Input: part model. Units: mm. Frame: model coordinates. A direction names the side the tool comes from. Coordinates: 2 decimals unless noted, no trailing zeros. Loops run counter-clockwise (first coordinate to the right, second up) from the corner with the lowest first, then second, coordinate; pieces in that order, holes last.
Autodesk Inventor part; units mm, degrees
ref_plane "YZ Plane" through (0, 0, 0) normal (1, 0, 0) x (0, 1, 0)
ref_plane "XZ Plane" through (0, 0, 0) normal (0, 1, 0) x (-1, 0, 0)
ref_plane "XY Plane" through (0, 0, 0) normal (0, 0, 1) x (1, 0, 0)
sketch "Sketch1" plane through (0, 0, 0) normal (0, 1, 0) x (-1, 0, 0)
  circle A0 centre (0, 0) radius 13.7
  dimension "d0" = 27.4
extrude "Extrusion1" add sketch "Sketch1" along normal blind 46.5
sketch "Sketch2" plane through (0, 46.5, 0) normal (0, 1, 0) x (1, 0, 0)
  circle A0 centre (0, 0) radius 13.7
  circle A1 centre (0, 0) radius 5
  dimension "d3" = 10
extrude "Extrusion2" add sketch "Sketch2" along normal blind 2.7 contours A1
sketch "Sketch3" plane through (0, 46.5, 0) normal (0, 1, 0) x (1, 0, 0)
  circle A0 centre (0, 0) radius 5
  circle A1 centre (0, 0) radius 5
  circle A2 centre (0, 0) radius 13.7
  circle A3 centre (0, 0) radius 13.7
  line L0 (-13.7, 0) -> (13.7, 0)
  point P0 (-8, 0)
  point P1 (8, 0)
  dimension "d6" = 16
  dimension "d7" = 5.7
  dimension "d8" = 5.7
hole "Hole1" at (-8, 46.5, 0) at (8, 46.5, 0) direction (0, -1, 0) diameter 2.1129 depth 2.8
ref_plane "Work Plane1" through (0, 41.5, 0) normal (0, 1, 0) x (1, 0, 0)
sketch "Sketch4" plane through (0, 41.5, 0) normal (0, 1, 0) x (1, 0, 0)
  circle A0 centre (0, 0) radius 14.375
  dimension "d17" = 28.75
extrude "Extrusion3" add sketch "Sketch4" against normal blind 27.7
sketch "Sketch5" plane through (0, 0, 0) normal (0, -1, 0) x (1, 0, 0)
  circle A0 centre (0, 0) radius 5
  dimension "d20" = 10
extrude "Extrusion4" add sketch "Sketch5" along normal blind 4
sketch "Sketch6" plane through (0, 0, 0) normal (0, -1, 0) x (1, 0, 0)
  circle A0 centre (0, 0) radius 5
  circle A1 centre (0, 0) radius 5
  circle A2 centre (0, 0) radius 13.7
  circle A3 centre (0, 0) radius 13.7
  line L0 (13.7, 0) -> (-13.7, 0)
  line L1 (-11.5, 1.5) -> (-12, 1.5)
  line L2 (-12, 1.5) -> (-12, -1.5)
  line L3 (-12, -1.5) -> (-11.5, -1.5)
  line L4 (-11.5, -1.5) -> (-11.5, 1.5)
  line L5 (11.5, 1.5) -> (11, 1.5)
  line L6 (11, 1.5) -> (11, -1.5)
  line L7 (11, -1.5) -> (11.5, -1.5)
  line L8 (11.5, -1.5) -> (11.5, 1.5)
  dimension "d23" = 22.5
  dimension "d24" = 0.5
  dimension "d25" = 0.5
  dimension "d26" = 11.5
  dimension "d27" = 11.5
  dimension "d28" = 3
  dimension "d29" = 3
  dimension "d30" = 1.5
  dimension "d31" = 1.5
extrude "Extrusion5" add sketch "Sketch6" along normal blind 6 contours L6 L5 L8 L0 | L0 L8 L7 L6 | L4 L3 L2 L0 | L0 L2 L1 L4
sketch "Sketch7" plane through (0, 49.2, 0) normal (0, 1, 0) x (1, 0, 0)
  circle A0 centre (0, 0) radius 1.1
  dimension "d34" = 2.2
extrude "Extrusion6" add sketch "Sketch7" along normal blind 13.5
sketch "Sketch8" plane through (0, 62.7, 0) normal (0, 1, 0) x (1, 0, 0)
  circle A0 centre (0, 0) radius 1.1
  circle A1 centre (0, 0) radius 5.925
  circle A2 centre (0, 0) radius 3.625
  circle A3 centre (0, 0) radius 4.775
  arc A4 (0.5843, 4.7391) -> (-0.5843, 4.7391) centre (0, 5.1881) ccw
  line L0 (0.4436, 3.5978) -> (0.725, 5.8805)
  line L1 (-0.4436, 3.5978) -> (-0.725, 5.8805)
  line L2 (-1.7559, 3.1714) -> (-2.8699, 5.1835)
  line L3 (-2.4736, 2.6499) -> (-4.043, 4.3313)
  arc A5 (-2.3129, 4.1775) -> (-3.2583, 3.4906) centre (-3.0495, 4.1973) ccw
  line L4 (-3.2846, 1.5336) -> (-5.3686, 2.5067)
  line L5 (-3.5587, 0.6899) -> (-5.8167, 1.1277)
  arc A6 (-4.3266, 2.0202) -> (-4.6877, 0.9088) centre (-4.9342, 1.6032) ccw
  line L6 (-3.5587, -0.6899) -> (-5.8167, -1.1277)
  line L7 (-3.2846, -1.5336) -> (-5.3686, -2.5067)
  arc A7 (-4.6877, -0.9088) -> (-4.3266, -2.0202) centre (-4.9342, -1.6032) ccw
  line L8 (-2.4736, -2.6499) -> (-4.043, -4.3313)
  line L9 (-1.7559, -3.1714) -> (-2.8699, -5.1835)
  arc A8 (-3.2583, -3.4906) -> (-2.3129, -4.1775) centre (-3.0495, -4.1973) ccw
  line L10 (-0.4436, -3.5978) -> (-0.725, -5.8805)
  line L11 (0.4436, -3.5978) -> (0.725, -5.8805)
  arc A9 (-0.5843, -4.7391) -> (0.5843, -4.7391) centre (0, -5.1881) ccw
  line L12 (1.7559, -3.1714) -> (2.8699, -5.1835)
  line L13 (2.4736, -2.6499) -> (4.043, -4.3313)
  arc A10 (2.3129, -4.1775) -> (3.2583, -3.4906) centre (3.0495, -4.1973) ccw
  line L14 (3.2846, -1.5336) -> (5.3686, -2.5067)
  line L15 (3.5587, -0.6899) -> (5.8167, -1.1277)
  arc A11 (4.3266, -2.0202) -> (4.6877, -0.9088) centre (4.9342, -1.6032) ccw
  line L16 (3.5587, 0.6899) -> (5.8167, 1.1277)
  line L17 (3.2846, 1.5336) -> (5.3686, 2.5067)
  arc A12 (4.6877, 0.9088) -> (4.3266, 2.0202) centre (4.9342, 1.6032) ccw
  line L18 (2.4736, 2.6499) -> (4.043, 4.3313)
  line L19 (1.7559, 3.1714) -> (2.8699, 5.1835)
  arc A13 (3.2583, 3.4906) -> (2.3129, 4.1775) centre (3.0495, 4.1973) ccw
  point P0 (3.7689, -4.0376)
  dimension "d37" = 11.85
  dimension "d38" = 7.25
  dimension "d39" = 1.45
  dimension "d43" = 1.15
  dimension "d44" = 1.15
  dimension "d47" = 360
extrude "Extrusion7" add sketch "Sketch8" along normal blind 5.5 and the other way blind 12.5 contours A12 L16 A3 L17 | A12 L16 | A11 L14 A3 L15 | L15 A11 | L17 A12 | L16 A2 L17 A3 | A11 L14 | A3 L14 A2 L15 | A2 | A13 L18 A3 L19 | A13 L18 | L18 A2 L19 A3 | A10 L12 A3 L13 | L13 A10 | A3 L12 A2 L13 | L19 A13 | A10 L12 | L0 A2 L1 A3 | L0 A4 | A3 L1 A4 L0 | L11 A9 L10 A3 | A3 L10 A2 L11 | A9 L11 | A4 L1 | L10 A9 | L2 A2 L3 A3 | A3 L3 A5 L2 | L2 A5 | L9 A8 L8 A3 | A3 L8 A2 L9 | A8 L9 | A5 L3 | L8 A8 | L4 A2 L5 A3 | A3 L5 A6 L4 | L4 A6 | L7 A7 L6 A3 | A3 L6 A2 L7 | A7 L7 | A6 L5 | L6 A7
equation "\"d26\" = d27"
equation "\"d30\" = d31"
equation "\"d43\" = d44"
equation "\"d41\" = d42"
properties part number "rs390" material "Steel, Mild"
Item 1: Section query A-A (y = 45). Output: boundary loops of the cut face in (x, z), then the cut area to 3 significant figures.
Result:
outline: circle Ø27.4 at (0, 0); hole circle Ø2.11 at (-8, 0); hole circle Ø2.11 at (8, 0)
area: 583 mm2
Item 2: Section query B-B (x = -8). Output: boundary loops of the cut face in (y, z).
Result:
outline: (0, -11.12) - (13.8, -11.12) - (13.8, -11.94) - (41.5, -11.94) - (41.5, -11.12) - (46.5, -11.12) - (46.5, -1.06) - (43.7, -1.06) - (43.7, 1.06) - (46.5, 1.06) - (46.5, 11.12) - (41.5, 11.12) - (41.5, 11.94) - (13.8, 11.94) - (13.8, 11.12) - (0, 11.12) - close
Item 3: Contact query for flat-ended pins moving along their axis: P1, Ø0.6, axis at x = -11.5, y = -1.5, coming from the -Z side; P2, Ø3, axis at x = 3.5, z = -4, coming from the -Y side; P3, Ø0.6, axis at x = -11.5, y = -1.5, coming from the +Z side. Output: stop coordinate, or through.
Result:
P1: stops at z = -1.5
P2: stops at y = -4
P3: stops at z = 1.5
Item 4: Mould query, pull axis Z, two halves, no side actions, for faces 5 (the face through (-5.64, 59.33, 1.81)), 6 (the face through (0, -4, 0)), 7 (the face through (-3.625, 59.326, -0.01)). Classes: +Z half, -Z half, draft (parallel to the pull), parting line (faces both ways), or undercut.
Result:
face 5: undercut
face 6: draft
face 7: undercut
Item 5: Reachability of faces 1 (the face through (-11.5, -3, 0)), 2 (the face through (13, 41.5, 5)), 3 (the face through (-0.1, 68.2, -1.4)), 4 (the face through (-12, -3, 0)) from +Z, -Z, +X, -X, +Y, -Y: full face, straight path, thin tool, end or side. Return the list, or none.
Result:
face 1: +Z, -Z, -Y
face 2: +Y
face 3: +Z, -Z, +X, -X, +Y
face 4: +Z, -Z, -X, -Y
Item 6: Section query D-D (y = 9.5). Output: boundary loops of the cut face in (x, z).
Result:
outline: circle Ø27.4 at (0, 0)
Item 7: Line query: L1, parallel to X at y = 45.4, z = 0; L2, parallel to Z at x = 0, y = 64.5; L3, parallel to Y at x = 1.75, z = -2.75. Output: solid intervals per line, ascending.
Result:
L1: x = -13.7 to -9.06, -6.94 to 6.94, 9.06 to 13.7
L2: z = -5.92 to -1.1, 1.1 to 5.92
L3: y = -4 to 49.2, 50.2 to 68.2
Item 8: Section query C-C (z = -8). Output: boundary loops of the cut face in (x, y).
Result:
outline: (-11.94, 13.8) - (-11.12, 13.8) - (-11.12, 0) - (11.12, 0) - (11.12, 13.8) - (11.94, 13.8) - (11.94, 41.5) - (11.12, 41.5) - (11.12, 46.5) - (-11.12, 46.5) - (-11.12, 41.5) - (-11.94, 41.5) - close
